Check sheet for the modelled part. Datum: model origin and axes. Units: mm. A direction names the side the tool comes from. Round coordinates to 2 decimals unless told otherwise and drop trailing zeros. Write each loop counter-clockwise with the first axis right and the second up, starting at its lowest first coordinate (ties: lowest second). Pieces come first, ordered by that corner, then holes. Notation, with made-up numbers: (-12.5, 73) -> (1.5, 73) arc R20 ccw to (1.5, 82) -> close; hole circle Ø6 at (-18, 21). An arc over 180 degrees is marked (long way). Put each result on its own line as item: value. Start each with the question number.
from build123d import *

# Parameters (mm, degrees)
F0_W      = 34
F0_H      = 34
F0_W_2    = 30
F0_H_2    = 30
F1_DEPTH  = 30
F2_W      = 32.414368
F2_H      = 32.092232
F3_DEPTH  = 1
F4_R      = 0.5
F5_DEPTH  = 2
F7_DEPTH  = 30
F10_DEPTH = 2


with BuildPart() as f1:
    # F0 (on Top) → F1 (new body)
    with BuildSketch(Plane.XY):
        with Locations((15, 15)):
            Rectangle(F0_W, F0_H)
        with Locations((15, 15)):
            Rectangle(F0_W_2, F0_H_2, mode=Mode.SUBTRACT)
    extrude(amount=F1_DEPTH)

    # F2 (on Top) → F3 (join)
    with BuildSketch(Plane.XY):
        with Locations((15.036923, 14.937822)):
            Rectangle(F2_W, F2_H)
    extrude(amount=F3_DEPTH)

    # F4 (on Top) → F5 (cut)
    with BuildSketch(Plane.XY):
        with Locations((15, 15)):
            Circle(F4_R)
    extrude(amount=F5_DEPTH, mode=Mode.SUBTRACT)

    # F6 (on Front) → F7 (join)
    with BuildSketch(Plane.XZ):
        Polygon((-2, 32.127354), (-2, 30), (-0.865411, 30), (0, 30), (0, 31.622646), (6.008863, 42.889264), (7.5, 42.889264), (9, 42.889264), (9, 45.016619), (7.5, 45.016619), (6.008863, 45.016619), (4.874274, 45.016619), align=None)
        Polygon((32, 32.127354), (25.125726, 45.016619), (23.991137, 45.016619), (22.5, 45.016619), (21, 45.016619), (21, 42.889264), (22.5, 42.889264), (23.991137, 42.889264), (29.999532, 31.623524), (29.999532, 30), (30.865411, 30), (32, 30), align=None)
    extrude(amount=-F7_DEPTH)

    # F9 (on offset) → F10 (cut)
    with BuildSketch(Plane.XY.offset(46)):
        Polygon((25.174274, 20.5), (4.874274, 20.5), (4.874274, 15), (4.874274, 9.5), (25.174274, 9.5), align=None)
    extrude(amount=-F10_DEPTH, mode=Mode.SUBTRACT)


solid = f1.part
1. Draft check along X on faces 1 (the cylindrical face through (14.935, 15.496, 0.493)), 2 (the flat face through (28.6, 14.8, 38.5)), 3 (the flat face through (15, -2, 15)), 4 (the flat face through (15, 0, 15)). Enter one of: released by +X, released by -X, zero draft, split by the parting line, or undercut.
2. Gauge pin test, flat ends, axial feed: P1, Ø6, axis at x = 16.5, y = 23, coming from the +Z side; P2, Ø1.1, axis at y = 18, z = 44, coming from the -X side; P3, Ø5.5, axis at x = 27.5, z = 41, coming from the -Y side. Record the tip position at first contact, or that the pin passes through.
3. Section check A-A, the plane x = 22. Enter the section's corners in (y, z).
4. Section check C-C, the plane x = 11. Enter the section's corners in (y, z).
5. Access from +Z, -Z, +X, -X, +Y, -Y to the whole of each face (thin tool, end or side, straight path). Record for faces 5 (the flat face through (27, 30, 39)), 6 (the flat face through (22, 15, 42.889)), 7 (the flat face through (11, 15, 1)), 8 (the flat face through (3, 0, 39)), 9 (the flat face through (21, 14.8, 43.7)).
6. Material ranges on L1, parallel to Y at x = 15, z = 0.5; L2, parallel to X at y = 26, z = 8.5, recorded low to high. Write a range as [from, to].
7. Section check B-B, the plane z = 20. Enter the section's corners in (x, y), then the cut area to 3 significant figures.
Reply:
1. face 1: undercut
1. face 2: released by +X
1. face 3: zero draft
1. face 4: undercut
2. P1: stops at z = 1
2. P2: stops at x = 4.04
2. P3: stops at y = 0
3. outline: (-2, 0) -> (32, 0) -> (32, 30) -> (30, 30) -> (30, 1) -> (0, 1) -> (0, 30) -> (-2, 30) -> close; (0, 42.89) -> (30, 42.89) -> (30, 45.02) -> (20.5, 45.02) -> (20.5, 44) -> (9.5, 44) -> (9.5, 45.02) -> (0, 45.02) -> close
4. outline: (-2, 0) -> (32, 0) -> (32, 30) -> (30, 30) -> (30, 1) -> (0, 1) -> (0, 30) -> (-2, 30) -> close
5. face 5: +Z, +X, -X, +Y
5. face 6: +Y, -Y
5. face 7: none
5. face 8: +Z, +X, -X, -Y
5. face 9: +Z, +Y, -Y
6. L1: y = [-2, 14.5], [15.5, 32]
6. L2: x = [-2, 0], [30, 32]
7. outline: (-2, -2) -> (32, -2) -> (32, 32) -> (-2, 32) -> close; hole (0, 0) -> (30, 0) -> (30, 30) -> (0, 30) -> close
7. area: 256 mm2
